```python
from build123d import *

# Parameters (mm, degrees)
CUT_EXTRUDE_2_DEPTH = 3


with BuildPart() as part:
    # 草图2 → 旋转1 (revolve)
    with BuildSketch(Plane(origin=(0, 0, 0), x_dir=(1, 0, 0), z_dir=(0, 1, 0))):
        Polygon((0, 0), (0, 8), (15, 8), (15, 9), (92, 9), (92, 11), (98, 11), (98, 9), (106, 9), (106, 0), align=None)
    revolve(axis=Axis((0, 0, 0), (1, 0, 0)))

    # 草图4 → 切除-拉伸2 (cut)
    with BuildSketch(Plane.XY.offset(9)):
        with BuildLine():
            Line((62, 3), (87, 3))
            ThreePointArc((87, 3), (90, 0), (87, -3))
            Line((87, -3), (62, -3))
            ThreePointArc((62, -3), (59, 0), (62, 3))
        make_face()
    extrude(amount=-CUT_EXTRUDE_2_DEPTH, mode=Mode.SUBTRACT)


solid = part.part
```
Part model, mm, in its own coordinate system. A direction names the side the tool comes from. Round coordinates to 2 decimals unless told otherwise and drop trailing zeros. Loops run counter-clockwise (first coordinate to the right, second up) from the corner with the lowest first, then second, coordinate; pieces in that order, holes last.
Item 1: Drop flat-ended pins along their axis: P1, Ø5, axis at x = 86.5, y = 2.5, coming from the +Z side; P2, Ø8, axis at x = 74, y = -8, coming from the +Z side; P3, Ø8, axis at x = 34.5, z = 3.5, coming from the -Y side; P4, Ø2, axis at y = -2.5, z = -5.5, coming from the -X side. Give the stop position or say it passes through.
Item 2: Cut at D-D, the plane x = 54. Give the cut face in (y, z).
Item 3: Cut at B-B, the plane y = 0. Give the cut face in (x, z).
Item 4: 3-axis set-ups, long thin cutter, end or side, ignore diameter. For faces 4 (the face through (0, 0, 0)), 5 (the face through (95.04, -10.74, 2.38)), 6 (the face through (98, -9, -2)), 7 (the face through (59, 0, 8)), 8 (the face through (54.039, 2.703, -8.584)): which of +Z, -Z, +X, -X, +Y, -Y reach the whole face in a straight line?
Item 5: Mould opens along Y. For faces 1 (the face through (92, -9, 2)), 2 (the face through (90, 0, 8)), 3 (the face through (7.6, -7.81, 1.73)) say: +Y half, -Y half, draft (parallel to the pull), parting line (faces both ways), or undercut.
Item 6: Drill centre lines: line 1 (Y direction, x = 20.5, z = -0.25); line 2 (X direction, y = 8.75, z = -4.75); line 3 (X direction, y = -6.5, z = -4.75). Where is each one in solid material? Low to high.
Item 7: Cut at C-C, the plane x = 78.5. Give the cut face in (y, z).
Item 8: Cut at A-A, the plane z = 0. Give the cut face in (x, y), then the cut area to 3 significant figures.
A:
1. P1: stops at z = 8.71
1. P2: stops at z = 8.06
1. P3: stops at y = -9
1. P4: stops at x = 0
2. outline: circle Ø18 at (0, 0)
3. outline: (0, -8) - (15, -8) - (15, -9) - (92, -9) - (92, -11) - (98, -11) - (98, -9) - (106, -9) - (106, 9) - (98, 9) - (98, 11) - (92, 11) - (92, 9) - (90, 9) - (90, 6) - (59, 6) - (59, 9) - (15, 9) - (15, 8) - (0, 8) - close
4. face 4: +Z, -Z, -X, +Y, -Y
4. face 5: +X, -X
4. face 6: +X
4. face 7: +Z
4. face 8: -X
5. face 1: draft
5. face 2: undercut
5. face 3: parting line
6. line 1: y = -9 to 9
6. line 2: x = 92 to 98
6. line 3: x = 15 to 106
7. outline: (-3, 6) - (-3, 8.49) arc R9 ccw (long way) to (3, 8.49) - (3, 6) - close
8. outline: (0, -8) - (15, -8) - (15, -9) - (92, -9) - (92, -11) - (98, -11) - (98, -9) - (106, -9) - (106, 9) - (98, 9) - (98, 11) - (92, 11) - (92, 9) - (15, 9) - (15, 8) - (0, 8) - close
8. area: 1,900 mm2
